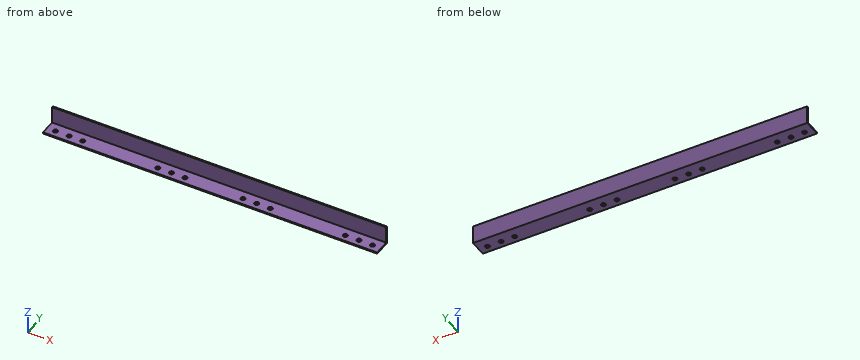
```python
from build123d import *

# Parameters (mm, degrees)
SKETCH_1_W        = 1960
SKETCH_1_H        = 100
SKETCH_1_R        = 13
EXTRUDE_708_DEPTH = 8
SKETCH_2_W        = 1960
SKETCH_2_H        = 8
EXTRUDE_1_DEPTH   = 100


with BuildPart() as part:
    # 草图1 → Extrude 708 (new body)
    with BuildSketch(Plane.XY):
        with Locations((0, 44.512115183)):
            Rectangle(SKETCH_1_W, SKETCH_1_H)
        with Locations((930, 34.512115183)):
            Circle(SKETCH_1_R, mode=Mode.SUBTRACT)
        with Locations((850, 34.512115183)):
            Circle(SKETCH_1_R, mode=Mode.SUBTRACT)
        with Locations((770, 34.512115183)):
            Circle(SKETCH_1_R, mode=Mode.SUBTRACT)
        with Locations((330, 34.512115183)):
            Circle(SKETCH_1_R, mode=Mode.SUBTRACT)
        with Locations((250, 34.512115183)):
            Circle(SKETCH_1_R, mode=Mode.SUBTRACT)
        with Locations(Location((-770, 34.512115183, 0), (0, 0, 180))):
            Circle(SKETCH_1_R, mode=Mode.SUBTRACT)
        with Locations(Location((-850, 34.512115183, 0), (0, 0, 180))):
            Circle(SKETCH_1_R, mode=Mode.SUBTRACT)
        with Locations((170, 34.512115183)):
            Circle(SKETCH_1_R, mode=Mode.SUBTRACT)
        with Locations(Location((-170, 34.512115183, 0), (0, 0, 180))):
            Circle(SKETCH_1_R, mode=Mode.SUBTRACT)
        with Locations(Location((-250, 34.512115183, 0), (0, 0, 180))):
            Circle(SKETCH_1_R, mode=Mode.SUBTRACT)
        with Locations(Location((-330, 34.512115183, 0), (0, 0, 180))):
            Circle(SKETCH_1_R, mode=Mode.SUBTRACT)
        with Locations(Location((-930, 34.512115183, 0), (0, 0, 180))):
            Circle(SKETCH_1_R, mode=Mode.SUBTRACT)
    extrude(amount=EXTRUDE_708_DEPTH)

    # 草图2 → 凸台-拉伸1 (add)
    with BuildSketch(Plane.XY.offset(8)):
        with Locations((0, 90.512115183)):
            Rectangle(SKETCH_2_W, SKETCH_2_H)
    extrude(amount=EXTRUDE_1_DEPTH)


solid = part.part
```
Check sheet for the modelled part. Datum: model origin and axes. Units: mm. Give positions to 0.01 mm unless a question says otherwise; leave off trailing zeros. Write each loop counter-clockwise with the first axis right and the second up, starting at its lowest first coordinate (ties: lowest second). Pieces come first, ordered by that corner, then holes.
Item 1: Scan lines: L1, parallel to Y at x = -770, z = 6.75; L2, parallel to Z at x = 91.5, y = 30; L3, parallel to Y at x = 572, z = 47. Record each from-to range of solid material in increasing order.
Item 2: Gauge pin test, flat ends, axial feed: pin 1 (21 mm diameter, centred on x = -850, y = 34.51, fed in from -Z); pin 2 (12 mm diameter, centred on x = 293, y = 7, fed in from +Z). Record the tip position at first contact, or that the pin passes through.
Item 3: Cross-section at A-A (x = 290). Enter the section's corners in (y, z).
Item 4: Cross-section at B-B (y = 70). Enter the section's corners in (x, z), and give its area (3 significant figures).
Item 5: Cross-section at C-C (z = 59.5). Enter the section's corners in (x, y), and give its area (3 significant figures).
Report:
1. L1: y = -5.49 to 21.51, 47.51 to 94.51
1. L2: z = 0 to 8
1. L3: y = 86.51 to 94.51
2. pin 1: passes through
2. pin 2: stops at z = 8
3. outline: (-5.49, 0) - (94.51, 0) - (94.51, 108) - (86.51, 108) - (86.51, 8) - (-5.49, 8) - close
4. outline: (-980, 0) - (980, 0) - (980, 8) - (-980, 8) - close
4. area: 15,700 mm2
5. outline: (-980, 86.51) - (980, 86.51) - (980, 94.51) - (-980, 94.51) - close
5. area: 15,700 mm2
